The drawing under review shows one solid part. Ordinate dimensions are in mm from its lowest x, y, z. Give positions to 0.01 mm unless a question says otherwise; leave off trailing zeros. Loops run counter-clockwise (first coordinate to the right, second up) from the corner with the lowest first, then second, coordinate; pieces in that order, holes last. Notation, with made-up numbers: M 89,43.25 L 126,43.25 A28 cw 126,62.25 Z; hole C -4,23 d2. An arc over 180 degrees is marked long. Write item = value, one per line. Start each with the question number.
1. We need section A-A on y = 33. Give the boundary of the cut face in (x, z) (1 decimal), then the cut area to 3 significant figures.
2. We need section C-C on x = 200. Give the boundary of the cut face in (y, z), then the cut area to 3 significant figures.
3. Wall thickness on line 1 along X through (y, z) = (44, 2.75) (1 decimal); line 2 along X through (y, z) = (68.5, 2.75) (1 decimal); line 3 along Y through (x, z) = (208, 7.25): over which ranges is each line inside the solid? List them lowest first. Write a range as from..to.
4. We need section B-B on z = 2.5. Give the boundary of the cut face in (x, y), then the cut area to 3 significant figures.
5. For pin 1 (3 mm diameter, centred on x = 163, y = 131, fed in from -Z); pin 2 (2 mm diameter, centred on x = 165, z = 3.5, fed in from -Y), all flat-tipped, find the tip position at first contact; note any pin that passes through.
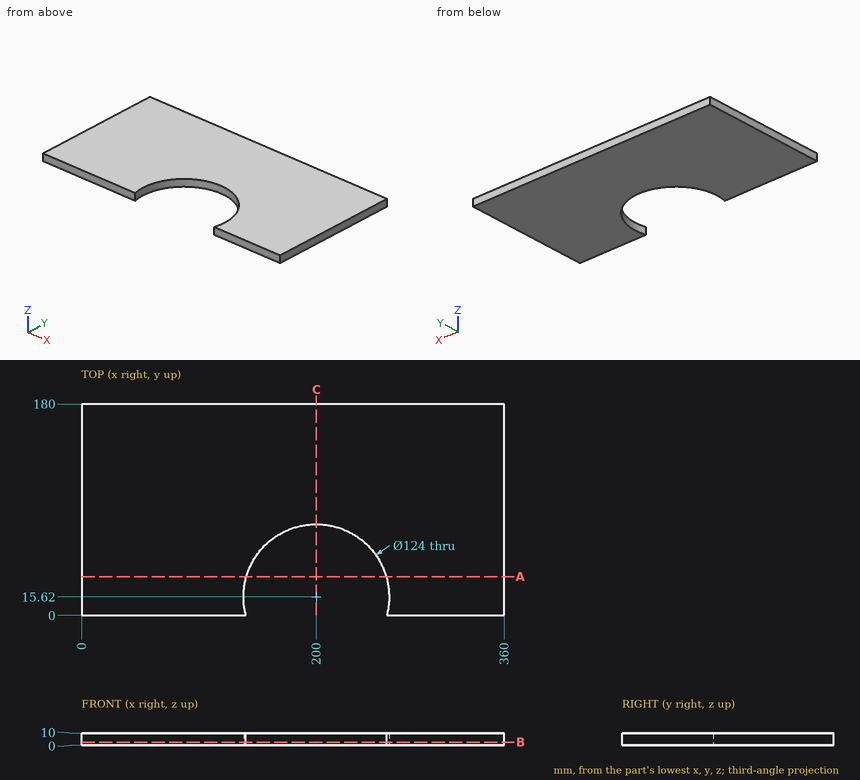
Final values:
q1.outline = M 0,0 L 140.5,0 L 140.5,10 L 0,10 Z; M 259.5,0 L 360,0 L 360,10 L 259.5,10 Z
q1.area = 2,410 mm²
q2.outline = M 77.62,0 L 180,0 L 180,10 L 77.62,10 Z
q2.area = 1,020 mm²
q3.line_1 = 0..144.9, 255.1..360
q3.line_2 = 0..167.6, 232.4..360
q3.line_3 = 77.1..180
q4.outline = M 0,0 L 140,0 A62 cw long 260,0 L 360,0 L 360,180 L 0,180 Z
q4.area = 56,800 mm²
q5.pin_1 = 0
q5.pin_2 = 66.1
